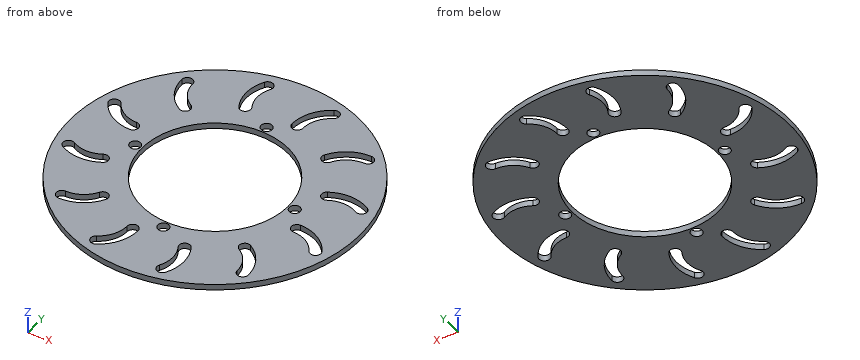
from build123d import *

# Parameters (mm, degrees)
SKETCH1_R           = 105
SKETCH1_R_2         = 53
SKETCH1_R_3         = 4
BOSS_EXTRUDE1_DEPTH = 4.25


with BuildPart() as part:
    # Sketch1 → Boss-Extrude1 (new body)
    with BuildSketch(Plane.XY):
        Circle(SKETCH1_R)
        Circle(SKETCH1_R_2, mode=Mode.SUBTRACT)
        with Locations((0, 58)):
            Circle(SKETCH1_R_3, mode=Mode.SUBTRACT)
        with Locations((58, 0)):
            Circle(SKETCH1_R_3, mode=Mode.SUBTRACT)
        with Locations((0, -58)):
            Circle(SKETCH1_R_3, mode=Mode.SUBTRACT)
        with Locations((-58, 0)):
            Circle(SKETCH1_R_3, mode=Mode.SUBTRACT)
        with BuildLine():
            ThreePointArc((94.5, 25.11473671), (80, 29), (65.5, 25.11473671))
            ThreePointArc((65.5, 25.11473671), (64.035898385, 19.650635095), (69.5, 18.186533479))
            ThreePointArc((69.5, 18.186533479), (80, 21), (90.5, 18.186533479))
            ThreePointArc((90.5, 18.186533479), (95.964101615, 19.650635095), (94.5, 25.11473671))
        make_face(mode=Mode.SUBTRACT)
        with BuildLine():
            ThreePointArc((94.396769013, -25.5), (83.782032303, -14.88526329), (69.282032303, -11))
            ThreePointArc((69.282032303, -11), (65.282032303, -15), (69.282032303, -19))
            ThreePointArc((69.282032303, -19), (79.782032303, -21.813466521), (87.468565782, -29.5))
            ThreePointArc((87.468565782, -29.5), (92.932667397, -30.964101615), (94.396769013, -25.5))
        make_face(mode=Mode.SUBTRACT)
        with BuildLine():
            ThreePointArc((69, -69.282032303), (65.11473671, -54.782032303), (54.5, -44.167295593))
            ThreePointArc((54.5, -44.167295593), (49.035898385, -45.631397208), (50.5, -51.095498823))
            ThreePointArc((50.5, -51.095498823), (58.186533479, -58.782032303), (61, -69.282032303))
            ThreePointArc((61, -69.282032303), (65, -73.282032303), (69, -69.282032303))
        make_face(mode=Mode.SUBTRACT)
        with BuildLine():
            ThreePointArc((25.11473671, -94.5), (29, -80), (25.11473671, -65.5))
            ThreePointArc((25.11473671, -65.5), (19.650635095, -64.035898385), (18.186533479, -69.5))
            ThreePointArc((18.186533479, -69.5), (21, -80), (18.186533479, -90.5))
            ThreePointArc((18.186533479, -90.5), (19.650635095, -95.964101615), (25.11473671, -94.5))
        make_face(mode=Mode.SUBTRACT)
        with BuildLine():
            ThreePointArc((-25.5, -94.396769013), (-14.88526329, -83.782032303), (-11, -69.282032303))
            ThreePointArc((-11, -69.282032303), (-15, -65.282032303), (-19, -69.282032303))
            ThreePointArc((-19, -69.282032303), (-21.813466521, -79.782032303), (-29.5, -87.468565782))
            ThreePointArc((-29.5, -87.468565782), (-30.964101615, -92.932667397), (-25.5, -94.396769013))
        make_face(mode=Mode.SUBTRACT)
        with BuildLine():
            ThreePointArc((-69.282032303, -69), (-54.782032303, -65.11473671), (-44.167295593, -54.5))
            ThreePointArc((-44.167295593, -54.5), (-45.631397208, -49.035898385), (-51.095498823, -50.5))
            ThreePointArc((-51.095498823, -50.5), (-58.782032303, -58.186533479), (-69.282032303, -61))
            ThreePointArc((-69.282032303, -61), (-73.282032303, -65), (-69.282032303, -69))
        make_face(mode=Mode.SUBTRACT)
        with BuildLine():
            ThreePointArc((-94.5, -25.11473671), (-80, -29), (-65.5, -25.11473671))
            ThreePointArc((-65.5, -25.11473671), (-64.035898385, -19.650635095), (-69.5, -18.186533479))
            ThreePointArc((-69.5, -18.186533479), (-80, -21), (-90.5, -18.186533479))
            ThreePointArc((-90.5, -18.186533479), (-95.964101615, -19.650635095), (-94.5, -25.11473671))
        make_face(mode=Mode.SUBTRACT)
        with BuildLine():
            ThreePointArc((-94.396769013, 25.5), (-83.782032303, 14.88526329), (-69.282032303, 11))
            ThreePointArc((-69.282032303, 11), (-65.282032303, 15), (-69.282032303, 19))
            ThreePointArc((-69.282032303, 19), (-79.782032303, 21.813466521), (-87.468565782, 29.5))
            ThreePointArc((-87.468565782, 29.5), (-92.932667397, 30.964101615), (-94.396769013, 25.5))
        make_face(mode=Mode.SUBTRACT)
        with BuildLine():
            ThreePointArc((-69, 69.282032303), (-65.11473671, 54.782032303), (-54.5, 44.167295593))
            ThreePointArc((-54.5, 44.167295593), (-49.035898385, 45.631397208), (-50.5, 51.095498823))
            ThreePointArc((-50.5, 51.095498823), (-58.186533479, 58.782032303), (-61, 69.282032303))
            ThreePointArc((-61, 69.282032303), (-65, 73.282032303), (-69, 69.282032303))
        make_face(mode=Mode.SUBTRACT)
        with BuildLine():
            ThreePointArc((-25.11473671, 94.5), (-29, 80), (-25.11473671, 65.5))
            ThreePointArc((-25.11473671, 65.5), (-19.650635095, 64.035898385), (-18.186533479, 69.5))
            ThreePointArc((-18.186533479, 69.5), (-21, 80), (-18.186533479, 90.5))
            ThreePointArc((-18.186533479, 90.5), (-19.650635095, 95.964101615), (-25.11473671, 94.5))
        make_face(mode=Mode.SUBTRACT)
        with BuildLine():
            ThreePointArc((25.5, 94.396769013), (14.88526329, 83.782032303), (11, 69.282032303))
            ThreePointArc((11, 69.282032303), (15, 65.282032303), (19, 69.282032303))
            ThreePointArc((19, 69.282032303), (21.813466521, 79.782032303), (29.5, 87.468565782))
            ThreePointArc((29.5, 87.468565782), (30.964101615, 92.932667397), (25.5, 94.396769013))
        make_face(mode=Mode.SUBTRACT)
        with BuildLine():
            ThreePointArc((69.282032303, 69), (54.782032303, 65.11473671), (44.167295593, 54.5))
            ThreePointArc((44.167295593, 54.5), (45.631397208, 49.035898385), (51.095498823, 50.5))
            ThreePointArc((51.095498823, 50.5), (58.782032303, 58.186533479), (69.282032303, 61))
            ThreePointArc((69.282032303, 61), (73.282032303, 65), (69.282032303, 69))
        make_face(mode=Mode.SUBTRACT)
    extrude(amount=BOSS_EXTRUDE1_DEPTH)


solid = part.part
Model file for the job. Use its own axes, mm. Round coordinates to 2 decimals unless told otherwise and drop trailing zeros. Order: outer loops, then holes, each group sorted by start corner. A loop starts at its lowest first (then second) coordinate and runs counter-clockwise, first axis right, second up.
(1) Band-saw the part on B-B (x = 58). List the corners of the cut face in (y, z), then the cut area to 3 significant figures.
(2) Band-saw the part on D-D (y = -37). List the corners of the cut face in (x, z).
(3) Band-saw the part on C-C (x = 15). List the corners of the cut face in (y, z).
(4) Pin check, flat tips, straight feed: pin 1 (1 mm diameter, centred on x = 49, z = 3.5, fed in from -Y); pin 2 (9 mm diameter, centred on x = 58, y = 0, fed in from -Z); pin 3 (1 mm diameter, centred on x = 32, z = 1.5, fed in from -Y). Stop position of each tip, or through.
(5) Band-saw the part on A-A (y = -14). List the corners of the cut face in (x, z), then the cut area to 3 significant figures.
(6) Drill centre lines: line 1 (Y direction, x = 0, z = 2.7); line 2 (X direction, y = -47, z = 0.45); line 3 (Y direction, x = -57, z = 2.6). Where is each one in solid material? Low to high.
Verdict:
1. outline: (-87.53, 0) - (-58.47, 0) - (-58.47, 4.25) - (-87.53, 4.25) - close; (-46.54, 0) - (-4, 0) - (-4, 4.25) - (-46.54, 4.25) - close; (4, 0) - (57.71, 0) - (57.71, 4.25) - (4, 4.25) - close; (66.72, 0) - (87.53, 0) - (87.53, 4.25) - (66.72, 4.25) - close
1. area: 621 mm2
2. outline: (-98.26, 0) - (-37.95, 0) - (-37.95, 4.25) - (-98.26, 4.25) - close; (37.95, 0) - (98.26, 0) - (98.26, 4.25) - (37.95, 4.25) - close
3. outline: (-103.92, 0) - (-50.83, 0) - (-50.83, 4.25) - (-103.92, 4.25) - close; (50.83, 0) - (65.28, 0) - (65.28, 4.25) - (50.83, 4.25) - close; (83.98, 0) - (103.92, 0) - (103.92, 4.25) - (83.98, 4.25) - close
4. pin 1: stops at y = -93.13
4. pin 2: stops at z = 0
4. pin 3: stops at y = -100.16
5. outline: (-104.06, 0) - (-51.12, 0) - (-51.12, 4.25) - (-104.06, 4.25) - close; (51.12, 0) - (65.41, 0) - (65.41, 4.25) - (51.12, 4.25) - close; (82.13, 0) - (104.06, 0) - (104.06, 4.25) - (82.13, 4.25) - close
5. area: 379 mm2
6. line 1: y = -105 to -62, -54 to -53, 53 to 54, 62 to 105
6. line 2: x = -93.89 to -24.49, 24.49 to 48.55, 58.56 to 93.89
6. line 3: y = -88.18 to -66.27, -57.03 to -3.87, 3.87 to 45.79, 56.95 to 88.18
